Part model, mm, in its own coordinate system. A direction names the side the tool comes from. Coordinates: 2 decimals unless noted, no trailing zeros. Loops run counter-clockwise (first coordinate to the right, second up) from the corner with the lowest first, then second, coordinate; pieces in that order, holes last. Notation, with made-up numbers: (57.5, -13.75) - (86.5, -13.75) arc R10 ccw to (86.5, -0.75) - close; hole circle Ø8 at (39, -6). An arc over 180 degrees is marked (long way). Use a Markdown table: item, result. Add a question column.
1) Probe probe 1 along Y at (x, z) = (0, 2.75); probe 2 along Y at (x, z) = (-6.5, 1); probe 3 along Z at (x, y) = (-4.25, -4.75). List the from-to ranges inside material, lowest first. Write a range as [from, to].
2) Band-saw the part on C-C (x = 1.75). Give the cut face in (y, z), plus the area to 3 significant figures.
3) Band-saw the part on A-A (x = 0). Give the cut face in (y, z).
4) Tool access for faces 1 (the face through (-1, -6, 4.5)), 2 (the face through (0, -14, 6)), 3 (the face through (-2, -11, 7)): list every direction of +Z, -Z, +X, -X, +Y, -Y with a clear straight run to the whole face (end or side of a thin tool).
5) Pull direction Y, two halves, no side cores. Call faces 4 (the face through (-6, 0.5, 4)), 5 (the face through (0, 5.5, 4)), 6 (the face through (0, -13, 12)): +Y half, -Y half, draft (parallel to the pull), parting line (faces both ways), or undercut.
6) Drop flat-ended pins along their axis: P1, Ø2, axis at x = -0.5, y = -13.5, coming from the -Z side; P2, Ø0.8, axis at y = -10.5, z = 6, coming from the -X side; P3, Ø1.1, axis at x = -5.5, z = 2, coming from the -Y side; P4, Ø1, axis at x = -4, z = 8.5, coming from the -Y side. Give the stop position or say it passes through.
7) Band-saw the part on D-D (y = -13). Give the cut face in (x, z).
8) Band-saw the part on B-B (y = -2). Give the cut face in (x, z), plus the area to 4 significant figures.
from build123d import *

# Parameters (mm, degrees)
EXTRUDE_1_DEPTH      = 7.5
FILLET_1_R           = 0.3
FILLET_2_R           = 1
HOLE_WIZARD_M3_1_D   = 2.5
SKETCH_4_W           = 4
SKETCH_4_H           = 5
EXTRUDE_2_DEPTH      = 2.5
SKETCH_5_W           = 4
SKETCH_5_H           = 6.5
EXTRUDE_3_DEPTH      = 1.5
FILLET_3_R           = 0.5
EXTRUDE_4_DEPTH      = 1
EXTRUDE_4_DEPTH_BACK = 1
FILLET_4_R           = 1
SKETCH_7_R           = 1.5
EXTRUDE_5_DEPTH      = 4.5


with BuildPart() as part:
    # 草图1 → 凸台-拉伸1 (new body)
    with BuildSketch(Plane.XY):
        with BuildLine():
            Line((-7.5, 0.5), (-7.5, -5.5))
            Line((-7.5, -5.5), (7.5, -5.5))
            Line((7.5, -5.5), (7.5, 0.5))
            Line((7.5, 0.5), (5, 0.5))
            ThreePointArc((5, 0.5), (3.5, 2), (5, 3.5))
            Line((5, 3.5), (7.5, 3.5))
            Line((7.5, 3.5), (7.5, 5.5))
            Line((7.5, 5.5), (-7.5, 5.5))
            Line((-7.5, 5.5), (-7.5, 3.5))
            Line((-7.5, 3.5), (-5, 3.5))
            ThreePointArc((-5, 3.5), (-3.5, 2), (-5, 0.5))
            Line((-5, 0.5), (-7.5, 0.5))
        make_face()
    extrude(amount=EXTRUDE_1_DEPTH)

    # 圆角1
    fillet_1_edges = [part.edges().sort_by_distance(p)[0] for p in [
        (7.5, 0.5, 3.75),
        (-7.5, 0.5, 3.75),
        (-7.5, 3.5, 3.75),
        (7.5, 3.5, 3.75),
    ]]
    fillet(fillet_1_edges, radius=FILLET_1_R)

    # 圆角2
    fillet_2_edges = [part.edges().sort_by_distance(p)[0] for p in [
        (7.5, -5.5, 3.75),
        (-7.5, -5.5, 3.75),
    ]]
    fillet(fillet_2_edges, radius=FILLET_2_R)

    # M3 螺纹孔1 (through all)
    with Locations(Plane(origin=(0, -2, 7.5), x_dir=(1, 0, 0), z_dir=(0, 0, 1))):
        with Locations((0, 0)):
            Hole(HOLE_WIZARD_M3_1_D / 2)

    # 草图4 → 凸台-拉伸2 (add)
    with BuildSketch(Plane.XY.offset(7.5)):
        with Locations((0, -8)):
            Rectangle(SKETCH_4_W, SKETCH_4_H)
    extrude(amount=-EXTRUDE_2_DEPTH)

    # 草图5 → 凸台-拉伸3 (add)
    with BuildSketch(Plane.XY.offset(7.5)):
        with Locations((0, -13.75)):
            Rectangle(SKETCH_5_W, SKETCH_5_H)
    extrude(amount=-EXTRUDE_3_DEPTH)

    # 圆角3
    fillet_3_edges = [part.edges().sort_by_distance(p)[0] for p in [
        (0, -10.5, 6),
    ]]
    fillet(fillet_3_edges, radius=FILLET_3_R)

    # 草图6 → 凸台-拉伸4 (add, two sides: drawn at the far end of the back side and taken through both)
    with BuildSketch(Plane.ZY.offset(-EXTRUDE_4_DEPTH_BACK)):
        Polygon((5, -7), (3.5, -5.5), (5, -5.5), align=None)
    extrude(amount=EXTRUDE_4_DEPTH + EXTRUDE_4_DEPTH_BACK)

    # 圆角4
    fillet_4_edges = [part.edges().sort_by_distance(p)[0] for p in [
        (0, -7, 5),
        (0, -5.5, 3.5),
        (-2, -5.5, 6.25),
        (2, -5.5, 6.25),
    ]]
    fillet(fillet_4_edges, radius=FILLET_4_R)

    # 草图7 → 凸台-拉伸5 (add)
    with BuildSketch(Plane.XY.offset(7.5)):
        with Locations((0, -13)):
            Circle(SKETCH_7_R)
    extrude(amount=EXTRUDE_5_DEPTH)


solid = part.part
Answer block:
| question | item | result |
|---|---|---|
| 1 | probe 1 | [-5.5, -3.25], [-0.75, 5.5] |
| 1 | probe 2 | [-5.5, 0.5], [3.5, 5.5] |
| 1 | probe 3 | [0, 7.5] |
| 2 | outline | (-17, 6) - (-11, 6) arc R0.5 cw to (-10.5, 5.5) - (-10.5, 5) - (-5.5, 5) - (-5.5, 0) - (5.5, 0) - (5.5, 7.5) - (-17, 7.5) - close |
| 2 | area | 105 mm2 |
| 3 | outline | (-17, 6) - (-11, 6) arc R0.5 cw to (-10.5, 5.5) - (-10.5, 5) - (-7.41, 5) arc R1 cw to (-6.71, 4.71) - (-5.79, 3.79) arc R1 cw to (-5.5, 3.09) - (-5.5, 0) - (-3.25, 0) - (-3.25, 7.5) - (-11.5, 7.5) - (-11.5, 12) - (-14.5, 12) - (-14.5, 7.5) - (-17, 7.5) - close; (-0.75, 0) - (5.5, 0) - (5.5, 7.5) - (-0.75, 7.5) - close |
| 4 | face 1 | -Z, -X, -Y |
| 4 | face 2 | -Z, +X, -X, -Y |
| 4 | face 3 | +Z, -Z, -X, -Y |
| 5 | face 4 | undercut |
| 5 | face 5 | +Y half |
| 5 | face 6 | draft |
| 6 | P1 | z = 6 |
| 6 | P2 | x = -2 |
| 6 | P3 | y = -5.5 |
| 6 | P4 | through |
| 7 | outline | (-2, 6) - (2, 6) - (2, 7.5) - (1.5, 7.5) - (1.5, 12) - (-1.5, 12) - (-1.5, 7.5) - (-2, 7.5) - close |
| 8 | outline | (-7.5, 0) - (-1.25, 0) - (-1.25, 7.5) - (-7.5, 7.5) - close; (1.25, 0) - (7.5, 0) - (7.5, 7.5) - (1.25, 7.5) - close |
| 8 | area | 93.75 mm2 |
